```python
from build123d import *

# Parameters (mm, degrees)
SKETCH1_W           = 114.3
SKETCH1_H           = 38.1
BOSS_EXTRUDE1_DEPTH = 6.35
CUT_EXTRUDE1_DEPTH  = 61.57513929


with BuildPart() as part:
    # Sketch1 → Boss-Extrude1 (new body)
    with BuildSketch(Plane.XY):
        Rectangle(SKETCH1_W, SKETCH1_H)
    extrude(amount=BOSS_EXTRUDE1_DEPTH)

    # Sketch2 → Cut-Extrude1 (cut, through all)
    with BuildSketch(Plane.XY.offset(6.35)):
        with BuildLine():
            Line((31.95195085, -1.58870754), (33.3375, -1.58870754))
            Line((33.3375, -1.58870754), (33.3375, 1.58629246))
            Line((33.3375, 1.58629246), (31.951327279, 1.58629246))
            ThreePointArc((31.951327279, 1.58629246), (44.449999878, 0.001247142), (31.95195085, -1.58870754))
        make_face()
        with BuildLine():
            Line((-32.057272724, 1.58870754), (-33.442821874, 1.58870754))
            Line((-33.442821874, 1.58870754), (-33.442821874, -1.58629246))
            Line((-33.442821874, -1.58629246), (-32.056649153, -1.58629246))
            ThreePointArc((-32.056649153, -1.58629246), (-44.555321751, -0.001247142), (-32.057272724, 1.58870754))
        make_face()
    extrude(amount=-CUT_EXTRUDE1_DEPTH, mode=Mode.SUBTRACT)


solid = part.part
```
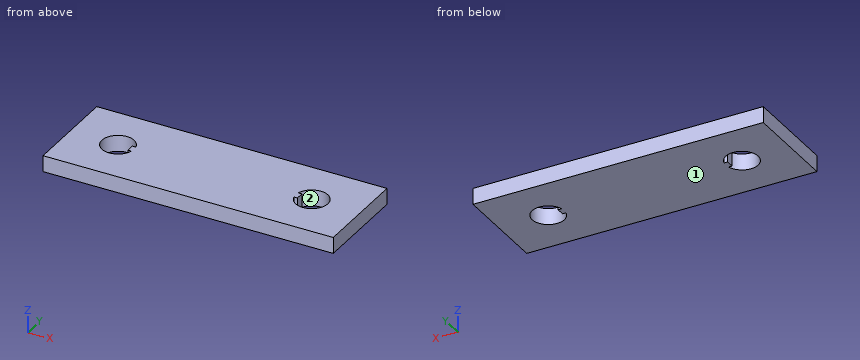
Here's how the part is built. I have some questions about the finished solid (model axes, mm). Face numbers are marked on the shaded views. Coordinates: 2 decimals unless noted, no trailing zeros. Write each loop counter-clockwise with the first axis right and the second up, starting at its lowest first coordinate (ties: lowest second). Pieces come first, ordered by that corner, then holes. Notation, with made-up numbers: (58.5, 28.5) -> (79.5, 28.5) arc R28 cw to (79.5, 46.5) -> close; hole circle Ø6 at (41, 46.25). An arc over 180 degrees is marked (long way). Use a Markdown table: item, result. Add a question column.
(1) I'm going to push a flat-ended pin straight in: P1, Ø1, axis at x = -18.5, y = 15, coming from the -Z side. Where does the tip first touch, or does it pass through?
(2) If we section it at D-D, the plane x = -35.5: Write out the boundary of the cut face in (y, z).
(3) If we section it at A-A, the plane x = 38.1: Write out the boundary of the cut face in (y, z), and give its area (3 significant figures).
(4) If we section it at B-B, the plane y = 0: Write out the boundary of the cut face in (x, z).
(5) If we section it at C-C, the plane z = 4.75: Write out the boundary of the cut face in (x, y).
(6) Please list where these lines run through material, in increasing order: line 1 (X direction, y = 0, z = 2.25); line 2 (X direction, y = -0.5, z = 3); line 3 (Y direction, x = 38.1, z = 3.75).
(7) We'd pull the mould along X, two halves only. Please class the marked faces 1 and 2: +X half, -X half, draft (parallel to the pull), parting line (faces both ways), or undercut.
Outcome:
| question | item | result |
|---|---|---|
| 1 | P1 | stops at z = 0 |
| 2 | outline | (-19.05, 0) -> (-5.74, 0) -> (-5.74, 6.35) -> (-19.05, 6.35) -> close; (5.74, 0) -> (19.05, 0) -> (19.05, 6.35) -> (5.74, 6.35) -> close |
| 3 | outline | (-19.05, 0) -> (-6.35, 0) -> (-6.35, 6.35) -> (-19.05, 6.35) -> close; (6.35, 0) -> (19.05, 0) -> (19.05, 6.35) -> (6.35, 6.35) -> close |
| 3 | area | 161 mm^2 |
| 4 | outline | (-57.15, 0) -> (-44.56, 0) -> (-44.56, 6.35) -> (-57.15, 6.35) -> close; (-33.44, 0) -> (33.34, 0) -> (33.34, 6.35) -> (-33.44, 6.35) -> close; (44.45, 0) -> (57.15, 0) -> (57.15, 6.35) -> (44.45, 6.35) -> close |
| 5 | outline | (-57.15, -19.05) -> (57.15, -19.05) -> (57.15, 19.05) -> (-57.15, 19.05) -> close; hole (-33.44, -1.59) -> (-33.44, 1.59) -> (-32.06, 1.59) arc R6.35 ccw (long way) to (-32.06, -1.59) -> close; hole (31.95, -1.59) arc R6.35 ccw (long way) to (31.95, 1.59) -> (33.34, 1.59) -> (33.34, -1.59) -> close |
| 6 | line 1 | x = -57.15 to -44.56, -33.44 to 33.34, 44.45 to 57.15 |
| 6 | line 2 | x = -57.15 to -44.54, -33.44 to 33.34, 44.43 to 57.15 |
| 6 | line 3 | y = -19.05 to -6.35, 6.35 to 19.05 |
| 7 | face 1 | draft |
| 7 | face 2 | undercut |
